The drawing under review shows one solid part. Ordinate dimensions are in mm from its lowest x, y, z. Give positions to 0.01 mm unless a question says otherwise; leave off trailing zeros. Loops run counter-clockwise (first coordinate to the right, second up) from the corner with the lowest first, then second, coordinate; pieces in that order, holes last. Notation, with made-up numbers: (71.25, 82.25) -> (101.25, 82.25) arc R16 cw to (101.25, 110.25) -> close; hole circle Ø5 at (38.5, -39). An arc over 180 degrees is marked (long way). Answer in a Markdown table with one row per item. Add a question column.
(1) For line 1 (Y direction, x = 35.5, z = 67); line 2 (Y direction, x = 34.5, z = 49.5), list the stretches that pass through material, from the lowest coordinate up.
(2) For pin 1 (1 mm diameter, centred on x = 14.5, z = 29.5, fed in from -Y), flat-tipped, find the tip position at first contact; note if it passes through.
(3) Consider section A-A on x = 9. Write out the cut boundary in (y, z), then the cut area to 3 significant figures.
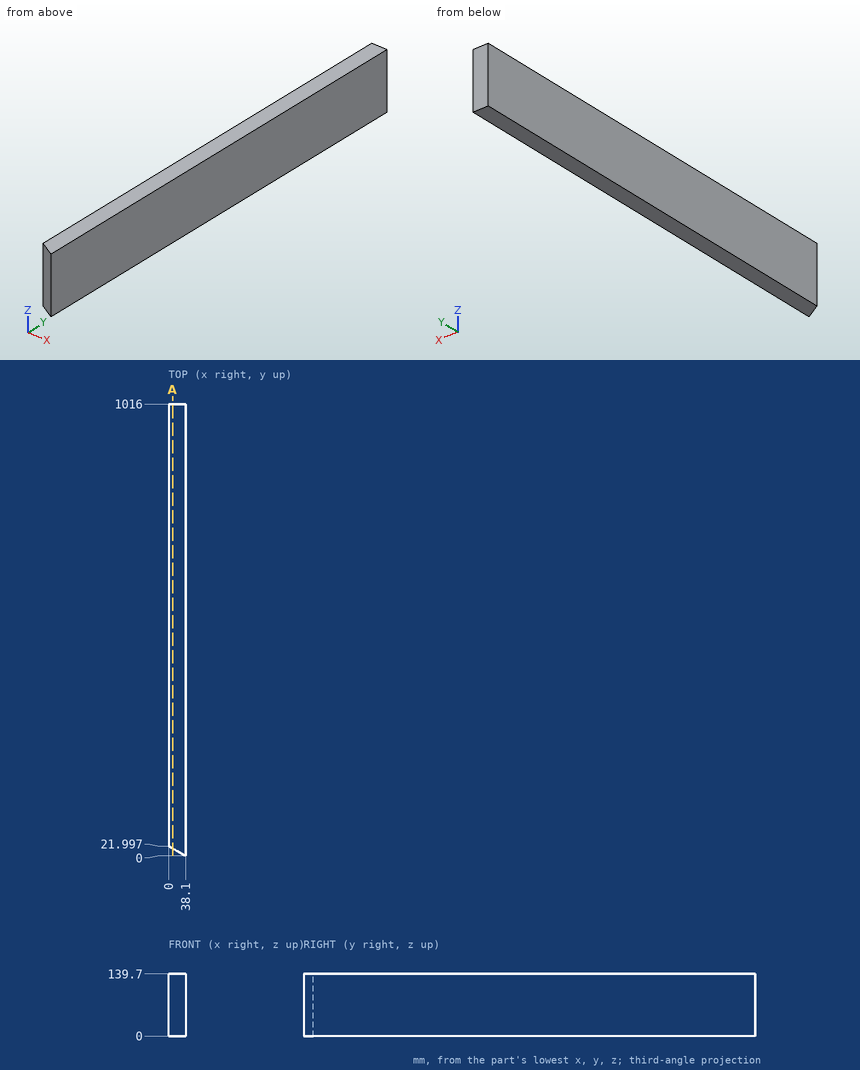
Values follow:
| question | item | result |
|---|---|---|
| 1 | line 1 | 1.5 to 1016 |
| 1 | line 2 | 2.08 to 1016 |
| 2 | pin 1 | y = 13.34 |
| 3 | outline | (16.8, 0) -> (1016, 0) -> (1016, 139.7) -> (16.8, 139.7) -> close |
| 3 | area | 140,000 mm2 |
